CAD build for the part. Positions are in the model's coordinates, mm. A direction names the side the tool comes from. Round coordinates to 2 decimals unless told otherwise and drop trailing zeros. Loops run counter-clockwise (first coordinate to the right, second up) from the corner with the lowest first, then second, coordinate; pieces in that order, holes last. Notation, with made-up numbers: M 54,-29.5 L 78,-29.5 A27 ccw 78,-2.5 Z; hole C -3.75,-15 d4. An arc over 180 degrees is marked long. Put each result on its own line as item: value. Start each with the question number.
from build123d import *

# Parameters (mm, degrees)
F1_DEPTH = 2.1
F3_DEPTH = 1.8
F5_DEPTH = 8


with BuildPart() as f1:
    # F0 (on Top) → F1 (new body)
    with BuildSketch(Plane.XY):
        Polygon((61.593626, -18.5), (61.593626, 18.5), (-25.406374, 18.5), (-25.406374, 30.5), (-47.352125, 0), (-25.406374, -30.5), (-25.406374, -18.5), align=None)
    extrude(amount=F1_DEPTH)

    # F2 (on face) → F3 (join)
    with BuildSketch(Plane.XY.offset(2.1)):
        Polygon((59.493628, 16.400002), (-27.506373, 16.400002), (-27.506373, 23.985889), (-44.765007, 0), (-27.506373, -23.985889), (-27.506373, -16.400002), (59.493628, -16.400002), align=None)
        Polygon((-29.606375, 17.471772), (-29.606375, 14.3), (57.393626, 14.3), (57.393626, -14.3), (-29.606375, -14.3), (-29.606375, -17.471772), (-42.177888, 0), align=None, mode=Mode.SUBTRACT)
    extrude(amount=F3_DEPTH)

    # F4 (on face) → F5 (cut)
    with BuildSketch(Plane.XY.offset(2.1)):
        Polygon((-7.031372, -2.5), (-7.031372, 0), (-7.031372, 2.5), (-17.031372, 2.5), (-17.031372, -2.5), align=None)
    extrude(amount=-F5_DEPTH, mode=Mode.SUBTRACT)


solid = f1.part
(1) Cut at A-A on z = 0.75. List the corners of the cut face in (x, y), and give its area (3 significant figures).
(2) Mould opens along X. For faces 6 (the flat face through (7, 0, 2.1)), 7 (the flat face through (-36.53, -15.04, 1.04)), 8 (the flat face through (6, 0, 0)) say: +X half, -X half, draft (parallel to the pull), parting line (faces both ways), or undercut.
(3) Drill centre lines: line 1 along Y through (x, z) = (7, 2.55); line 2 along Y through (x, z) = (29.5, 1.9); line 3 along Z through (x, y) = (-32, 0). Where is each one in solid material? Low to high.
(4) Flat gauge pins, fed straight in: pin 1 Ø1.7 at (x, z) = (-14, 1) entering from -Y; pin 2 Ø0.5 at (y, z) = (-16.5, 3.5) entering from -X; pin 3 Ø1.7 at (y, z) = (26, 1) entering from +X. Where does each tip first touch, or does it go through?
(5) Tool access for faces 1 (the flat face through (-35.98, 8.614, 2.987)), 2 (the flat face through (19, 18.5, 1)), 3 (the flat face through (-17.031, 0, 1)), 4 (the flat face through (-36.257, -11.825, 2.987)), 5 (the flat face through (17, -18.5, 1)): list every direction of +Z, -Z, +X, -X, +Y, -Y with a clear straight run to the whole face (end or side of a thin tool).
(6) Cut at B-B on y = 19.5. List the corners of the cut face in (x, z), and give its area (3 significant figures).
(7) Cut at D-D on x = -35.5. List the corners of the cut face in (y, z).
(8) Cut at C-C on x = 8. List the corners of the cut face in (y, z).
Taken from the geometry:
1. outline: M -47.35,0 L -25.41,-30.5 L -25.41,-18.5 L 61.59,-18.5 L 61.59,18.5 L -25.41,18.5 L -25.41,30.5 Z; hole M -17.03,-2.5 L -7.03,-2.5 L -7.03,2.5 L -17.03,2.5 Z
1. area: 3,840 mm2
2. face 6: undercut
2. face 7: -X half
2. face 8: draft
3. line 1: -16.4 to -14.3, 14.3 to 16.4
3. line 2: -18.5 to 18.5
3. line 3: 0 to 2.1
4. pin 1: y = -18.5
4. pin 2: x = -33.07
4. pin 3: x = -25.41
5. face 1: +Z
5. face 2: +Z, -Z, +X, +Y
5. face 3: +Z, -Z
5. face 4: +Z, -X, -Y
5. face 5: +Z, -Z, +X, -Y
6. outline: M -33.32,0 L -25.41,0 L -25.41,2.1 L -27.51,2.1 L -27.51,3.9 L -30.73,3.9 L -30.73,2.1 L -33.32,2.1 Z
6. area: 22.4 mm2
7. outline: M -16.47,0 L 16.47,0 L 16.47,2.1 L 12.88,2.1 L 12.88,3.9 L 9.28,3.9 L 9.28,2.1 L -9.28,2.1 L -9.28,3.9 L -12.88,3.9 L -12.88,2.1 L -16.47,2.1 Z
8. outline: M -18.5,0 L 18.5,0 L 18.5,2.1 L 16.4,2.1 L 16.4,3.9 L 14.3,3.9 L 14.3,2.1 L -14.3,2.1 L -14.3,3.9 L -16.4,3.9 L -16.4,2.1 L -18.5,2.1 Z
